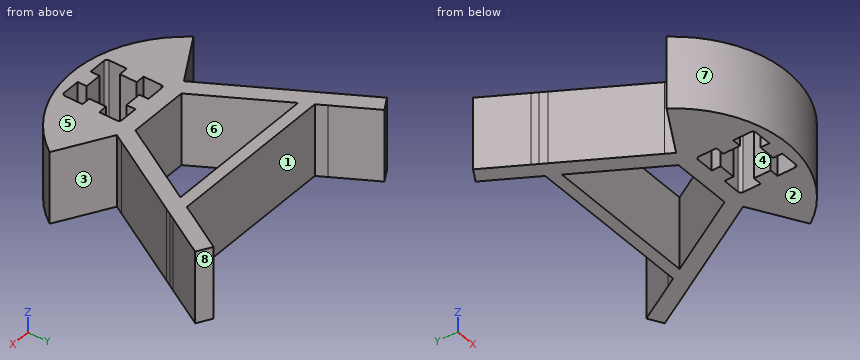
from build123d import *

# Parameters (mm, degrees)
F0_W     = 3.1
F0_H     = 2.9
F0_W_2   = 2.9
F0_H_2   = 3.1
F1_DEPTH = 25
F2_R     = 1


with BuildPart() as f1:
    # F0 (on Top) → F1 (new body)
    with BuildSketch(Plane.XY):
        with BuildLine():
            Line((-10, -0.3823358958), (-32.44, -0.3823358958))
            ThreePointArc((-32.44, -0.3823358958), (0, -17.2338951597), (32.44, -0.3823358958))
            Line((32.44, -0.3823358958), (10, -0.3823358958))
            Line((10, -0.3823358958), (10, -0.4138951597))
            Line((10, -0.4138951597), (10, -3.3138951597))
            Line((10, -3.3138951597), (10, -6.2138951597))
            Line((10, -6.2138951597), (10, -13.3138951597))
            Line((10, -13.3138951597), (2.9, -13.3138951597))
            Line((2.9, -13.3138951597), (0, -13.3138951597))
            Line((0, -13.3138951597), (-2.9, -13.3138951597))
            Line((-2.9, -13.3138951597), (-10, -13.3138951597))
            Line((-10, -13.3138951597), (-10, -6.2138951597))
            Line((-10, -6.2138951597), (-10, -3.3138951597))
            Line((-10, -3.3138951597), (-10, -0.4138951597))
            Line((-10, -0.4138951597), (-10, -0.3823358958))
        make_face()
        with BuildLine():
            Line((28.8595280896, 44.4161048403), (32.9867018661, 44.4161048403))
            ThreePointArc((32.9867018661, 44.4161048403), (31.8657182591, 46.010563932), (30.6677337786, 47.5480089641))
            Line((30.6677337786, 47.5480089641), (28.8595280896, 44.4161048403))
        make_face()
        with BuildLine():
            Line((32.9867018661, 44.4161048403), (35.2103810507, 44.4161048403))
            Line((35.2103810507, 44.4161048403), (43.2644919243, 58.3662340832))
            Line((43.2644919243, 58.3662340832), (38.5013522035, 61.1162340832))
            Line((38.5013522035, 61.1162340832), (30.6677337786, 47.5480089641))
            ThreePointArc((30.6677337786, 47.5480089641), (31.8657182591, 46.010563932), (32.9867018661, 44.4161048403))
        make_face()
        with BuildLine():
            Line((-35.2103810507, 44.4161048403), (-32.9867018661, 44.4161048403))
            ThreePointArc((-32.9867018661, 44.4161048403), (-31.8657182591, 46.010563932), (-30.6677337786, 47.5480089641))
            Line((-30.6677337786, 47.5480089641), (-38.5013522035, 61.1162340832))
            Line((-38.5013522035, 61.1162340832), (-43.2644919243, 58.3662340832))
            Line((-43.2644919243, 58.3662340832), (-35.2103810507, 44.4161048403))
        make_face()
        with BuildLine():
            ThreePointArc((-30.6677337786, 47.5480089641), (-31.8657182591, 46.010563932), (-32.9867018661, 44.4161048403))
            Line((-32.9867018661, 44.4161048403), (-28.8595280896, 44.4161048403))
            Line((-28.8595280896, 44.4161048403), (-30.6677337786, 47.5480089641))
        make_face()
        Polygon((-15.1194919243, 9.6176641042), (-32.44, -0.3823358958), (-10, -0.3823358958), (-10, 6.6861048403), (-2.9, 6.6861048403), (0, 6.6861048403), (2.9, 6.6861048403), (10, 6.6861048403), (10, -0.3823358958), (32.44, -0.3823358958), (15.1194919243, 9.6176641042), (10.3563522035, 12.3676641042), (10.3843194756, 12.4161048403), (-10.3843194756, 12.4161048403), (-10.3563522035, 12.3676641042), align=None)
        Polygon((10.3563522035, 12.3676641042), (15.1194919243, 9.6176641042), (16.7351724366, 12.4161048403), (10.3843194756, 12.4161048403), align=None)
        Polygon((-16.7351724366, 12.4161048403), (-15.1194919243, 9.6176641042), (-10.3563522035, 12.3676641042), (-10.3843194756, 12.4161048403), align=None)
        with Locations((-8.45, -4.7638951597)):
            Rectangle(F0_W, F0_H)
        with Locations((-8.45, -1.8638951597)):
            Rectangle(F0_W, F0_H)
        with Locations((-1.45, 5.1361048403)):
            Rectangle(F0_W_2, F0_H_2)
        with Locations((1.45, 5.1361048403)):
            Rectangle(F0_W_2, F0_H_2)
        with Locations((8.45, -4.7638951597)):
            Rectangle(F0_W, F0_H)
        with Locations((8.45, -1.8638951597)):
            Rectangle(F0_W, F0_H)
        with Locations((1.45, -11.7638951597)):
            Rectangle(F0_W_2, F0_H_2)
        with Locations((-1.45, -11.7638951597)):
            Rectangle(F0_W_2, F0_H_2)
        Polygon((-32.900979974, 40.4161048403), (-16.7351724366, 12.4161048403), (-10.3843194756, 12.4161048403), (-26.5501270129, 40.4161048403), align=None)
        Polygon((-28.8595280896, 44.4161048403), (-26.5501270129, 40.4161048403), (26.5501270129, 40.4161048403), (28.8595280896, 44.4161048403), align=None)
        with BuildLine():
            Line((26.5501270129, 40.4161048403), (32.900979974, 40.4161048403))
            Line((32.900979974, 40.4161048403), (34.1452121911, 42.5711782568))
            ThreePointArc((34.1452121911, 42.5711782568), (33.5786302545, 43.501599623), (32.9867018661, 44.4161048403))
            Line((32.9867018661, 44.4161048403), (28.8595280896, 44.4161048403))
            Line((28.8595280896, 44.4161048403), (26.5501270129, 40.4161048403))
        make_face()
        Polygon((10.3843194756, 12.4161048403), (16.7351724366, 12.4161048403), (32.900979974, 40.4161048403), (26.5501270129, 40.4161048403), align=None)
        with BuildLine():
            Line((-34.1452121911, 42.5711782568), (-32.900979974, 40.4161048403))
            Line((-32.900979974, 40.4161048403), (-26.5501270129, 40.4161048403))
            Line((-26.5501270129, 40.4161048403), (-28.8595280896, 44.4161048403))
            Line((-28.8595280896, 44.4161048403), (-32.9867018661, 44.4161048403))
            ThreePointArc((-32.9867018661, 44.4161048403), (-33.5786302545, 43.501599623), (-34.1452121911, 42.5711782568))
        make_face()
        with BuildLine():
            Line((-35.2103810507, 44.4161048403), (-34.1452121911, 42.5711782568))
            ThreePointArc((-34.1452121911, 42.5711782568), (-33.5786302545, 43.501599623), (-32.9867018661, 44.4161048403))
            Line((-32.9867018661, 44.4161048403), (-35.2103810507, 44.4161048403))
        make_face()
        with BuildLine():
            ThreePointArc((32.9867018661, 44.4161048403), (33.5786302545, 43.501599623), (34.1452121911, 42.5711782568))
            Line((34.1452121911, 42.5711782568), (35.2103810507, 44.4161048403))
            Line((35.2103810507, 44.4161048403), (32.9867018661, 44.4161048403))
        make_face()
    extrude(amount=F1_DEPTH)

    # F2
    f2_edges = [f1.edges().sort_by_distance(p)[0] for p in [
        (-10, -13.313895, 12.5),
        (-10, 6.686105, 12.5),
        (10, -13.313895, 12.5),
        (10, 6.686105, 12.5),
    ]]
    fillet(f2_edges, radius=F2_R)


solid = f1.part
Check sheet for the modelled part. Datum: model origin and axes. Units: mm. Face numbers are marked on the shaded views. A direction names the side the tool comes from. Coordinates: 2 decimals unless noted, no trailing zeros. Write each loop counter-clockwise with the first axis right and the second up, starting at its lowest first coordinate (ties: lowest second). Pieces come first, ordered by that corner, then holes. Notation, with made-up numbers: M 73.5,38 L 81.5,38 A31 ccw 81.5,64 Z; hole C 65.25,63.25 d10. An arc over 180 degrees is marked long. Answer as CSV lines item,"result".
Q1. Cross-section at A-A (y = 27.5). Record the boundary of the cut face in (x, z).
Check result:
outline,"M -25.44,0 L -19.09,0 L -19.09,25 L -25.44,25 Z; M 19.09,0 L 25.44,0 L 25.44,25 L 19.09,25 Z"
Q2. Cross-section at B-B (x = -13). Record the boundary of the cut face in (y, z), then the cut area to 3 significant figures.
Check result:
outline,"M -15.04,0 L 16.95,0 L 16.95,25 L -15.04,25 Z; M 40.42,0 L 44.42,0 L 44.42,25 L 40.42,25 Z"
area,"900 mm^2"
Q3. Set-up check for the marked faces 1, 2, 3 and 4: record each of +Z, -Z, +X, -X, +Y, -Y from which the full face is reachable in a straight line by a thin tool's end or side.
Check result:
face 1,"+Z, -Z, +Y"
face 2,"-Z, +X, -X, +Y, -Y"
face 3,"+Z, -Z, +X"
face 4,"+Z, -Z"
Q4. Cross-section at C-C (x = 5). Record the boundary of the cut face in (y, z), then the cut area to 3 significant figures.
Check result:
outline,"M -16.92,0 L -13.31,0 L -13.31,25 L -16.92,25 Z; M 6.69,0 L 12.42,0 L 12.42,25 L 6.69,25 Z; M 40.42,0 L 44.42,0 L 44.42,25 L 40.42,25 Z"
area,"333 mm^2"
Q5. Cross-section at D-D (z = 23). Count the separate pieces of the cut face and the enclosed holes in it, then the cut area to 3 significant figures.
Check result:
separate pieces,"1"
enclosed holes,"2"
area,"1,830 mm^2"
Q6. Go/stop test with flat-tipped pins: pin 1 (3 mm diameter, centred on x = -7, z = 18, fed in from -Y); pin 2 (7.5 mm diameter, centred on x = 4, z = 13, fed in from -Y); pin 3 (10 mm diameter, centred on y = 31, z = 8.5, fed in from +X); pin 4 (5 mm diameter, centred on x = -24, y = 48.5, fed in from -Z). Record where each tip stops, or that it passes through.
Check result:
pin 1,"y = -16.85"
pin 2,"y = -17.23"
pin 3,"x = 30.35"
pin 4,"through"
Q7. Material ranges on probe 1 along Y at (x, z) = (-24.5, 3.5); probe 2 along X at (y, z) = (-10.5, 7.5); probe 3 along Y at (x, z) = (8, 11), recorded low to high. Write a range as from..to.
Check result:
probe 1,"-8.76..4.2, 25.87..36.87, 40.42..44.42"
probe 2,"-22.11..-10, -2.9..2.9, 10..22.11"
probe 3,"-16.42..-13.31, -6.21..-0.41, 6.69..12.42, 40.42..44.42"
Q8. Mould release check, pull along Y, two halves, no side actions. Record for the marked faces 5, 6, 7 and 8: released by +Y, released by -Y, zero draft, split by the parting line, or undercut.
Check result:
face 5,"zero draft"
face 6,"undercut"
face 7,"released by -Y"
face 8,"released by +Y"
